Design review of the part built by this model. Coordinates are the model's own, in mm. Face numbers are marked on the shaded views. A direction names the side the tool comes from. Coordinates: 2 decimals unless noted, no trailing zeros. Loops run counter-clockwise (first coordinate to the right, second up) from the corner with the lowest first, then second, coordinate; pieces in that order, holes last. Notation, with made-up numbers: (3.5, -18.5) -> (11.5, -18.5) arc R21 cw to (11.5, 4.5) -> close; hole circle Ø4 at (-10, -7.5). An arc over 180 degrees is marked (long way). Answer as a JSON object with one key per item and string values.
```python
from build123d import *

# Parameters (mm, degrees)
F0_R     = 25.4
F0_W     = 12.7
F0_H     = 12.7
F1_DEPTH = 50.8
F2_W     = 13.873184
F2_H     = 11.720448
F3_DEPTH = 50.8
F4_W     = 13.275202
F4_H     = 13.394801
F5_DEPTH = 50.8


with BuildPart() as f1:
    # F0 (on Front) → F1 (new body)
    with BuildSketch(Plane.XZ):
        with Locations((-6.32722, 8.622332)):
            Circle(F0_R)
        with Locations((-6.32722, 8.622332)):
            Rectangle(F0_W, F0_H, mode=Mode.SUBTRACT)
    extrude(amount=F1_DEPTH)

    # F2 (on Right) → F3 (cut, symmetric)
    with BuildSketch(Plane.YZ):
        with Locations((-23.919283, 9.089327)):
            Rectangle(F2_W, F2_H)
    extrude(amount=F3_DEPTH, both=True, mode=Mode.SUBTRACT)

    # F4 (on Top) → F5 (cut, symmetric)
    with BuildSketch(Plane.XY):
        with Locations((-6.637601, -23.68009)):
            Rectangle(F4_W, F4_H)
    extrude(amount=F5_DEPTH, both=True, mode=Mode.SUBTRACT)


solid = f1.part
```
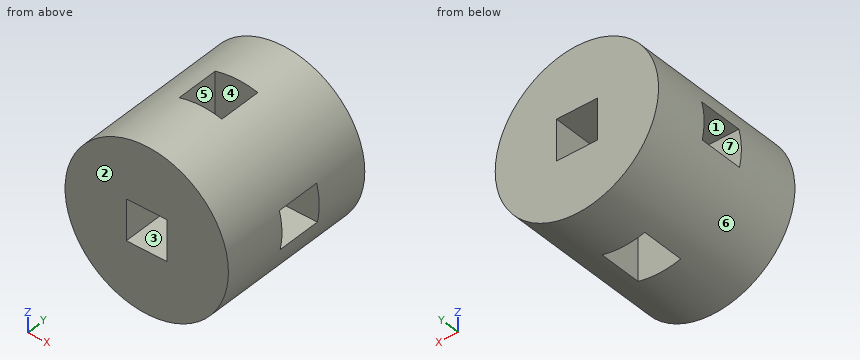
1) Clearance check with flat-ended pins moving along their axes: pin 1 Ø3 at (x, y) = (-15.5, -17) entering from +Z; pin 2 Ø8 at (y, z) = (-44.5, 16.5) entering from -X; pin 3 Ø14 at (x, y) = (-3.5, -35) entering from -Z; pin 4 Ø4 at (x, z) = (-6, 26.5) entering from +Y. State where each tip first meets the part, or that it passes through.
Completed:
{"pin 1": "z = 32.84", "pin 2": "x = -31.43", "pin 3": "z = -16.78", "pin 4": "y = 0"}
2) Add section C-C, the plane x = 7. Give the boundary of the cut face in (y, z), and give its area (3 significant figures).
Completed:
{"outline": "(-50.8, -13) -> (0, -13) -> (0, 30.25) -> (-50.8, 30.25) -> close; hole (-30.86, 3.23) -> (-16.98, 3.23) -> (-16.98, 14.95) -> (-30.86, 14.95) -> close", "area": "2,030 mm²"}
3) Add section A-A, the plane x = -11. Give the boundary of the cut face in (y, z), and give its area (3 significant figures).
Completed:
{"outline": "(-50.8, -16.34) -> (-30.38, -16.34) -> (-30.38, 2.27) -> (-50.8, 2.27) -> close; (-50.8, 14.97) -> (-30.38, 14.97) -> (-30.38, 33.59) -> (-50.8, 33.59) -> close; (-16.98, -16.34) -> (0, -16.34) -> (0, 2.27) -> (-16.98, 2.27) -> close; (-16.98, 14.97) -> (0, 14.97) -> (0, 33.59) -> (-16.98, 33.59) -> close", "area": "1,390 mm²"}
4) Add section B-B, the plane z = 12.5. Count the separate pieces of the cut face and the enclosed holes in it, and give its area (3 significant figures).
Completed:
{"separate pieces": "4", "enclosed holes": "0", "area": "1,380 mm²"}
5) Add section D-D, the plane z = 28.5. Give the boundary of the cut face in (x, y).
Completed:
{"outline": "(-22.14, -50.8) -> (9.49, -50.8) -> (9.49, 0) -> (-22.14, 0) -> close; hole (-13.28, -30.38) -> (0, -30.38) -> (0, -16.98) -> (-13.28, -16.98) -> close"}
6) Wall thickness on probe 1 along X at (y, z) = (-37, 14); probe 2 along Y at (x, z) = (-0.5, 30.5); probe 3 along Y at (x, z) = (14, 5): over which ranges is each line inside the solid? List them lowest first.
Completed:
{"probe 1": "-31.15 to -12.68, 0.02 to 18.5", "probe 2": "-50.8 to -30.38, -16.98 to 0", "probe 3": "-50.8 to -30.86, -16.98 to 0"}
7) The part is to be moulded in two halves that separate along X. For the marked faces 5, 6 and 7, say which applies: pulls with the +X half, pulls with the -X half, needs draft (parallel to the pull), parting line crosses it, or undercut.
Completed:
{"face 5": "undercut", "face 6": "parting line crosses it", "face 7": "needs draft"}
8) For the marked faces 1, 2, 3 and 4, list the 3-axis set-ups (+Z, -Z, +X, -X, +Y, -Y) from which the entire face can be reached by the end or side of a thin tool; tool diameter is ignored.
Completed:
{"face 1": "+X, -X", "face 2": "+Z, -Z, +X, -X, -Y", "face 3": "+Y, -Y", "face 4": "+Z, -Z"}
